Read the model definition and answer for the solid it produces. Units are mm, in the model's axes. A direction names the side the tool comes from. Coordinates: 2 decimals unless noted, no trailing zeros. Write each loop counter-clockwise with the first axis right and the second up, starting at its lowest first coordinate (ties: lowest second). Pieces come first, ordered by that corner, then holes. Notation, with made-up numbers: (67.25, -22.75) -> (83.25, -22.75) arc R34 cw to (83.25, 7.25) -> close; hole circle Ø10 at (-12.75, -3). An arc over 180 degrees is marked (long way). Use CSV: the item, a comma, the result in double quotes. Start each with the question number.
from build123d import *

# Parameters (mm, degrees)
SKETCH1_R           = 3.175
SKETCH1_R_2         = 3.2639
SKETCH1_R_3         = 2.6289
SKETCH1_R_4         = 2.0193
BOSS_EXTRUDE1_DEPTH = 6.35
SKETCH2_R           = 3.175
CUT_EXTRUDE1_DEPTH  = 0.79375


with BuildPart() as part:
    # Sketch1 → Boss-Extrude1 (new body)
    with BuildSketch(Plane.XY):
        with BuildLine():
            Line((159.591131024, -50.8), (268.282803213, -50.8))
            ThreePointArc((268.282803213, -50.8), (268.798556268, 47.996235774), (234.123018172, 140.508771477))
            Line((234.123018172, 140.508771477), (152.715190262, 152.715190262))
            Line((152.715190262, 152.715190262), (118.427127597, 118.427127597))
            ThreePointArc((118.427127597, 118.427127597), (154.732498954, 64.092299607), (167.48125, 0))
            ThreePointArc((167.48125, 0), (165.496965553, -25.70454229), (159.591131024, -50.8))
        make_face()
        with Locations((176.898422575, 6.177429038)):
            Circle(SKETCH1_R, mode=Mode.SUBTRACT)
        with Locations((144.995031539, 101.526614087)):
            Circle(SKETCH1_R, mode=Mode.SUBTRACT)
        with Locations((163.532451502, 67.7373593)):
            Circle(SKETCH1_R, mode=Mode.SUBTRACT)
        with Locations((172.12665951, -41.275)):
            Circle(SKETCH1_R, mode=Mode.SUBTRACT)
        with Locations((193.675, 0)):
            Circle(SKETCH1_R_2, mode=Mode.SUBTRACT)
        with Locations((219.075, 0)):
            Circle(SKETCH1_R_2, mode=Mode.SUBTRACT)
        with Locations((215.746758491, 38.041974522)):
            Circle(SKETCH1_R_2, mode=Mode.SUBTRACT)
        with Locations((190.732641565, 33.63131081)):
            Circle(SKETCH1_R_2, mode=Mode.SUBTRACT)
        with Locations((205.863160899, 74.928062899)):
            Circle(SKETCH1_R_2, mode=Mode.SUBTRACT)
        with Locations((181.994968331, 66.240751259)):
            Circle(SKETCH1_R_2, mode=Mode.SUBTRACT)
        with Locations((189.724515334, 109.5375)):
            Circle(SKETCH1_R_2, mode=Mode.SUBTRACT)
        with Locations((167.727470078, 96.8375)):
            Circle(SKETCH1_R_2, mode=Mode.SUBTRACT)
        with Locations((167.821186376, 140.818695592)):
            Circle(SKETCH1_R_2, mode=Mode.SUBTRACT)
        with Locations((148.363657521, 124.491890306)):
            Circle(SKETCH1_R_2, mode=Mode.SUBTRACT)
        with Locations((263.525, 0)):
            Circle(SKETCH1_R_2, mode=Mode.SUBTRACT)
        with Locations((254.545603373, 68.205288861)):
            Circle(SKETCH1_R_2, mode=Mode.SUBTRACT)
        with Locations((228.219344532, 131.7625)):
            Circle(SKETCH1_R_2, mode=Mode.SUBTRACT)
        with Locations((240.38178065, 21.030680725)):
            Circle(SKETCH1_R, mode=Mode.SUBTRACT)
        with Locations((233.077901884, 62.453035583)):
            Circle(SKETCH1_R, mode=Mode.SUBTRACT)
        with Locations((218.692069012, 101.977786558)):
            Circle(SKETCH1_R, mode=Mode.SUBTRACT)
        with Locations((228.6, -38.1)):
            Circle(SKETCH1_R_3, mode=Mode.SUBTRACT)
        with Locations((254, -38.1)):
            Circle(SKETCH1_R_3, mode=Mode.SUBTRACT)
        with Locations((159.651941396, 76.436052669)):
            Circle(SKETCH1_R_4, mode=Mode.SUBTRACT)
        with Locations((139.323763183, 109.179217581)):
            Circle(SKETCH1_R_4, mode=Mode.SUBTRACT)
        with Locations((176.974598028, -3.347266353)):
            Circle(SKETCH1_R_4, mode=Mode.SUBTRACT)
        with Locations((174.097718528, -31.956172212)):
            Circle(SKETCH1_R_4, mode=Mode.SUBTRACT)
        with BuildLine():
            Line((202.565, 0), (202.565, 9.525))
            ThreePointArc((202.565, 9.525), (206.375, 13.335), (210.185, 9.525))
            Line((210.185, 9.525), (210.185, 0))
            Line((210.185, 0), (210.185, -9.525))
            ThreePointArc((210.185, -9.525), (206.375, -13.335), (202.565, -9.525))
            Line((202.565, -9.525), (202.565, 0))
        make_face(mode=Mode.SUBTRACT)
        with BuildLine():
            Line((199.487582489, 35.175043109), (201.141581381, 25.794749262))
            ThreePointArc((201.141581381, 25.794749262), (205.555298477, 22.70423128), (208.645816459, 27.117948375))
            Line((208.645816459, 27.117948375), (206.991817567, 36.498242223))
            Line((206.991817567, 36.498242223), (205.337818675, 45.87853607))
            ThreePointArc((205.337818675, 45.87853607), (200.924101579, 48.969054052), (197.833583597, 44.555336957))
            Line((197.833583597, 44.555336957), (199.487582489, 35.175043109))
        make_face(mode=Mode.SUBTRACT)
        with BuildLine():
            Line((190.348835729, 69.281310333), (193.606577595, 60.33073812))
            ThreePointArc((193.606577595, 60.33073812), (198.489903226, 58.053605981), (200.767035365, 62.936931612))
            Line((200.767035365, 62.936931612), (197.5092935, 71.887503825))
            Line((197.5092935, 71.887503825), (194.251551635, 80.838076038))
            ThreePointArc((194.251551635, 80.838076038), (189.368226003, 83.115208177), (187.091093864, 78.231882546))
            Line((187.091093864, 78.231882546), (190.348835729, 69.281310333))
        make_face(mode=Mode.SUBTRACT)
        with BuildLine():
            Line((175.426435918, 101.2825), (180.188935918, 93.033608029))
            ThreePointArc((180.188935918, 93.033608029), (185.393492706, 91.639051241), (186.788049494, 96.843608029))
            Line((186.788049494, 96.843608029), (182.025549494, 105.0925))
            Line((182.025549494, 105.0925), (177.263049494, 113.341391971))
            ThreePointArc((177.263049494, 113.341391971), (172.058492706, 114.735948759), (170.663935918, 109.531391971))
            Line((170.663935918, 109.531391971), (175.426435918, 101.2825))
        make_face(mode=Mode.SUBTRACT)
        with BuildLine():
            Line((155.17379262, 130.206272156), (161.296344603, 122.909698835))
            ThreePointArc((161.296344603, 122.909698835), (166.663994724, 122.4400903), (167.133603259, 127.807740421))
            Line((167.133603259, 127.807740421), (161.011051277, 135.104313742))
            Line((161.011051277, 135.104313742), (154.888499295, 142.400887063))
            ThreePointArc((154.888499295, 142.400887063), (149.520849174, 142.870495598), (149.051240638, 137.502845477))
            Line((149.051240638, 137.502845477), (155.17379262, 130.206272156))
        make_face(mode=Mode.SUBTRACT)
    extrude(amount=BOSS_EXTRUDE1_DEPTH)

    # Sketch2 → Cut-Extrude1 (cut)
    with BuildSketch(Plane.XY.offset(6.35)):
        with Locations((202.565, 0)):
            Circle(SKETCH2_R)
        with Locations((210.185, 0)):
            Circle(SKETCH2_R)
        with Locations((199.487582489, 35.175043109)):
            Circle(SKETCH2_R)
        with Locations((206.991817567, 36.498242223)):
            Circle(SKETCH2_R)
        with Locations((190.348835729, 69.281310333)):
            Circle(SKETCH2_R)
        with Locations((197.5092935, 71.887503825)):
            Circle(SKETCH2_R)
        with Locations((175.426435918, 101.2825)):
            Circle(SKETCH2_R)
        with Locations((182.025549494, 105.0925)):
            Circle(SKETCH2_R)
        with Locations((155.17379262, 130.206272156)):
            Circle(SKETCH2_R)
        with Locations((161.011051277, 135.104313742)):
            Circle(SKETCH2_R)
    extrude(amount=-CUT_EXTRUDE1_DEPTH, mode=Mode.SUBTRACT)


solid = part.part
1) Find the intervals of material crossed by line 1 along X through (y, z) = (64.5, 5.5); line 2 along Y through (x, z) = (178.5, 0.75); line 3 along Y through (x, z) = (189.5, 6), in increasing order.
2) The mould has two halves that part along Y. Classify faces 1 (the face through (175.36, 101.4, 3.13)), 2 (the face through (213, -50.8, 3)), 3 (the face through (212, 52, 0)): pulls with the +Y half, pulls with the -Y half, needs draft (parallel to the pull), parting line crosses it, or undercut.
3) Section B-B, the plane z = 1.5 is taken. Count the separate pieces of the cut face and the enclosed holes in it, plus the area to 3 significant figures.
4) Each of these flat-tipped pins is pushed along its axis until it touches: pin 1 (7.5 mm diameter, centred on x = 167.73, y = 96.84, fed in from +Z); pin 2 (1.9 mm diameter, centred on y = 4, z = 4.5, fed in from -X); pin 3 (1 mm diameter, centred on y = 43.5, z = 5.5, fed in from -X); pin 4 (3 mm diameter, centred on y = 82.5, z = 5.5, fed in from +X). Where does it stop, or does it pass through?
5) Section A-A, the plane x = 254 is taken. Give the vertices of the cut face in (y, z), plus the area to 3 significant figures.
6) Which of the six approach directions +Z, -Z, +X, -X, +Y, -Y give full straight-line access (tool end or side, diameter ignored) to faces 4 (the face through (174, 100, 5.556)), 5 (the face through (257.561, 66.955, 3.131))?
The answers:
1,line 1,"x = 154.56 to 179.23, 184.76 to 192.09, 200.2 to 230.65, 235.5 to 265.32"
1,line 2,"y = -50.8 to -4.67, -2.02 to 3.44, 8.92 to 95.96, 111.2 to 148.85"
1,line 3,"y = -50.8 to 30.61, 36.65 to 66.22, 83.16 to 106.28, 112.79 to 147.2"
2,face 1,"undercut"
2,face 2,"pulls with the -Y half"
2,face 3,"needs draft"
3,separate pieces,"1"
3,enclosed holes,"31"
3,area,"20,000 mm^2"
4,pin 1,"stops at z = 6.35"
4,pin 2,"stops at x = 167.41"
4,pin 3,"stops at x = 161.6"
4,pin 4,"stops at x = 260.76"
5,outline,"(-50.8, 0) -> (-40.73, 0) -> (-40.73, 6.35) -> (-50.8, 6.35) -> close; (-35.47, 0) -> (64.99, 0) -> (64.99, 6.35) -> (-35.47, 6.35) -> close; (71.42, 0) -> (100.2, 0) -> (100.2, 6.35) -> (71.42, 6.35) -> close"
5,area,"885 mm^2"
6,face 4,"+Z"
6,face 5,"+Z, -Z"
